The model under review builds one solid part; all positions refer to its coordinate system, in mm. A direction names the side the tool comes from. Give positions to 0.01 mm unless a question says otherwise; leave off trailing zeros. Order: outer loops, then holes, each group sorted by start corner. A loop starts at its lowest first (then second) coordinate and runs counter-clockwise, first axis right, second up. Notation, with made-up numbers: (54, 51) -> (78, 51) arc R29 cw to (78, 84) -> close; hole circle Ø2 at (85.25, 75.5). An arc over 180 degrees is marked (long way). Answer as a JSON object with one key per item and string values. Group by question number.
from build123d import *

# Parameters (mm, degrees)
F1_DEPTH = 14.224


with BuildPart() as f1:
    # F0 (on Front) → F1 (new body)
    with BuildSketch(Plane.XZ):
        Polygon((4.784628, 39.629921), (-4.784628, 39.629921), (-4.784628, -39.629921), (-2.392314, -39.629921), (0, -39.629921), (2.392314, -39.629921), (4.784628, -39.629921), align=None)
        Polygon((0, -39.629921), (-2.392314, -39.629921), (-2.392314, -95.287018), (-1.196157, -99.425659), (-0.598078, -97.356338), (0, -95.287018), (0.598078, -97.356338), (1.196157, -99.425659), (2.392314, -95.287018), (2.392314, -39.629921), align=None)
        Polygon((0, -95.287018), (-0.598078, -97.356338), (0, -99.425659), (0.598078, -97.356338), align=None)
    extrude(amount=F1_DEPTH)


solid = f1.part
1. For probe 1 along Z at (x, y) = (3, -10.5); probe 2 along X at (y, z) = (-4.25, -44.5), list the stretches that pass through material, from the lowest coordinate up. Write a range as [from, to].
2. Machinability: for faces 1 (the flat face through (2.392, -7, -68)), 2 (the flat face through (-2.392, -7, -67)), 3 (the flat face through (0, -14.224, -13)), which of the approach directions +Z, -Z, +X, -X, +Y, -Y give a long, thin tool a straight path to every point of the face, cutting with its end or side? Answer none if there is none.
3. For pin 1 (1.2 mm diameter, centred on x = -3.5, y = -9.5, fed in from -Z); pin 2 (7 mm diameter, centred on y = -5.5, z = -66.5, fed in from -X), all flat-tipped, find the tip position at first contact; note any pin that passes through.
4. Take a section at A-A on y = -3. Give the boundary of the cut face in (x, z), plus the area to 3 significant figures.
5. Take a section at B-B on z = -56.5. Give the boundary of the cut face in (x, y).
Checks:
{
 "1": {"probe 1": "z = [-39.63, 39.63]", "probe 2": "x = [-2.39, 2.39]"},
 "2": {"face 1": "-Z, +X, +Y, -Y", "face 2": "-Z, -X, +Y, -Y", "face 3": "+Z, -Z, +X, -X, -Y"},
 "3": {"pin 1": "stops at z = -39.63", "pin 2": "stops at x = -2.39"},
 "4": {"outline": "(-4.78, -39.63) -> (-2.39, -39.63) -> (-2.39, -95.29) -> (-1.2, -99.43) -> (-0.6, -97.36) -> (0, -99.43) -> (0.6, -97.36) -> (1.2, -99.43) -> (2.39, -95.29) -> (2.39, -39.63) -> (4.78, -39.63) -> (4.78, 39.63) -> (-4.78, 39.63) -> close", "area": "1,040 mm2"},
 "5": {"outline": "(-2.39, -14.22) -> (2.39, -14.22) -> (2.39, 0) -> (-2.39, 0) -> close"}
}
